Job drawing, mm, ordinate dimensions from the low corner. One solid piece. A direction names the side the tool comes from. Round coordinates to 2 decimals unless told otherwise and drop trailing zeros. Write each loop counter-clockwise with the first axis right and the second up, starting at its lowest first coordinate (ties: lowest second). Pieces come first, ordered by that corner, then holes. Notation, with made-up numbers: (63, 54.25) - (84, 54.25) arc R16 cw to (84, 77.25) - close; hole circle Ø5 at (-35.5, 18.5). An arc over 180 degrees is marked (long way). Write each question's results on one line, items separated by ' | '.
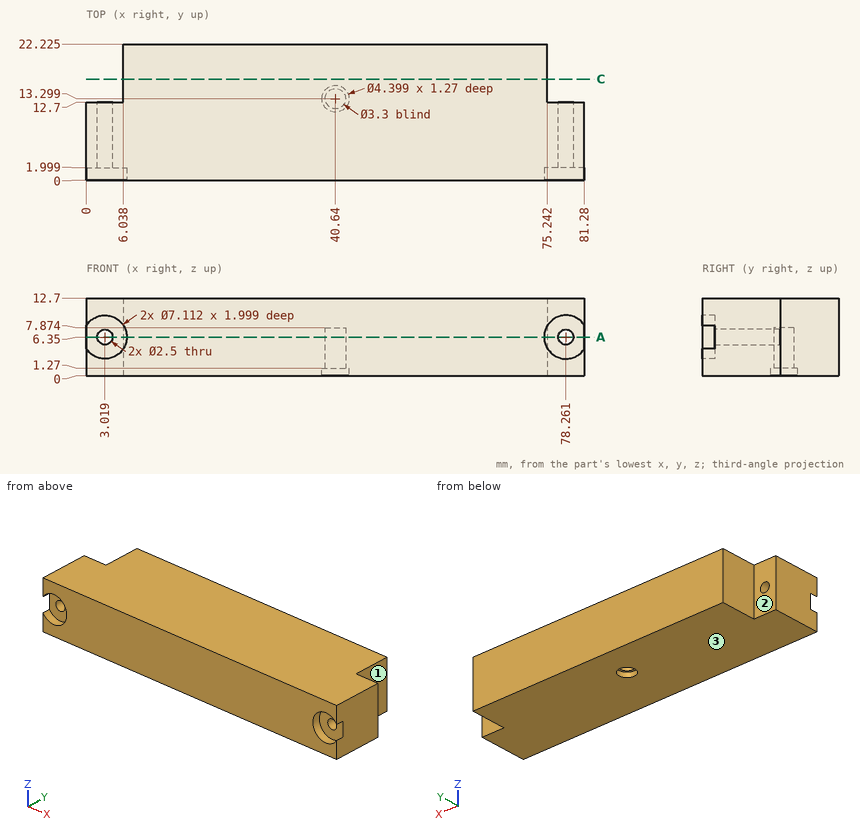
(1) Flat gauge pins, fed straight in: pin 1 Ø7.5 at (y, z) = (16.5, 8) entering from +X; pin 2 Ø5 at (x, z) = (3.5, 8) entering from +Y; pin 3 Ø4.5 at (x, z) = (78.26, 6.35) entering from -Y. Where does each tip first touch, or does it go through?
Worked answers:
pin 1: stops at x = 75.24 | pin 2: stops at y = 12.7 | pin 3: stops at y = 2
(2) Slice it at A-A, the plane z = 6.35. State how many separate pieces and enclosed holes the cut face has, and give its area (3 significant figures).
Worked answers:
separate pieces: 3 | enclosed holes: 1 | area: 1,600 mm2
(3) Drill centre lines: probe 1 along X at (y, z) = (5.25, 6.35); probe 2 along Y at (x, z) = (40.64, 0.95) (1 decimal); probe 3 along X at (y, z) = (1.4, 6.35) (1 decimal). Where is each one in solid material? Low to high. Write a range as [from, to].
Worked answers:
probe 1: x = [0, 1.77], [4.27, 77.01], [79.51, 81.28] | probe 2: y = [0, 11.1], [15.5, 22.2] | probe 3: x = [6.6, 74.7]
(4) Tool access for the marked faces 1, 2 and 3: list every direction of +Z, -Z, +X, -X, +Y, -Y with a clear straight run to the whole face (end or side of a thin tool).
Worked answers:
face 1: +Z, -Z, +X, +Y | face 2: +Z, -Z, -X, +Y | face 3: -Z, +X, -X, +Y, -Y
(5) Slice it at C-C, the plane y = 16.5. Write the cut outline in (x, z).
Worked answers:
outline: (6.04, 0) - (75.24, 0) - (75.24, 12.7) - (6.04, 12.7) - close
